Source: CAD feature listing. Evaluate the final solid. Frame: model axes, mm. Round coordinates to 2 decimals unless told otherwise and drop trailing zeros. Order: outer loops, then holes, each group sorted by start corner. A loop starts at its lowest first (then second) coordinate and runs counter-clockwise, first axis right, second up. Notation, with made-up numbers: (72.5, -25.75) - (124.5, -25.75) arc R18 ccw to (124.5, -0.75) - close; hole circle Ø11 at (35.25, 48). An arc over 180 degrees is marked (long way). Put each result on its own line as item: value. Start each with the question number.
1) Section A-A on z = 42.5. Output: boundary loops of the cut face in (x, y), then the cut area to 3 significant figures.
2) Section B-B on x = 5.25. Output: boundary loops of the cut face in (y, z), then the cut area to 3 significant figures.
3) Section C-C on y = 32. Output: boundary loops of the cut face in (x, z), then the cut area to 3 significant figures.
4) Line query: probe 1 along Z at (x, y) = (4.5, 0); probe 2 along Y at (x, z) = (5.25, 46.5); probe 3 along Z at (x, y) = (1.25, 37). Output: solid intervals per line, ascending. Write a range as [from, to].
```python
from build123d import *

# Parameters (mm, degrees)
F1_DEPTH = 10


with BuildPart() as f1:
    # F0 (on Right) → F1 (new body)
    with BuildSketch(Plane.YZ):
        Polygon((86, -121.5), (86, 121.5), (0, 121.5), (-86, 121.5), (-86, -121.5), align=None)
        with BuildLine():
            ThreePointArc((41.5, 46.5), (-29.344931, 17.155069), (0, 88))
            ThreePointArc((0, 88), (29.344931, 75.844931), (41.5, 46.5))
        make_face(mode=Mode.SUBTRACT)
    extrude(amount=F1_DEPTH)


solid = f1.part
```
Answer sheet:
1. outline: (0, -86) - (10, -86) - (10, -41.31) - (0, -41.31) - close; (0, 41.31) - (10, 41.31) - (10, 86) - (0, 86) - close
1. area: 894 mm^2
2. outline: (-86, -121.5) - (86, -121.5) - (86, 121.5) - (-86, 121.5) - close; hole (0, 88) arc R41.5 ccw (long way) to (41.5, 46.5) arc R41.5 ccw to start
2. area: 36,400 mm^2
3. outline: (0, -121.5) - (10, -121.5) - (10, 20.08) - (0, 20.08) - close; (0, 72.92) - (10, 72.92) - (10, 121.5) - (0, 121.5) - close
3. area: 1,900 mm^2
4. probe 1: [-121.5, 5], [88, 121.5]
4. probe 2: [-86, -41.5], [41.5, 86]
4. probe 3: [-121.5, 27.71], [65.29, 121.5]
